Geometry: final body of the model. Coordinates: model frame, mm. Face numbers are marked on the shaded views. Give positions to 0.01 mm unless a question says otherwise; leave off trailing zeros. One line per question, with ' | ' between items. Start each with the question number.
Item 1: Pin query (flat end, axial travel): P1, Ø12, axis at x = 53.5, z = -242, coming from the +Y side; P2, Ø1.5, axis at x = 238.5, z = -43.5, coming from the -Y side. Return the tip coordinate at first contact, or that it passes through.
Item 2: Section A-A on y = 2.55. Give the number of separate pieces and of enclosed holes in the cut face, then the cut area to 3 significant figures.
Item 3: Material intervals for line 1 along X through (y, z) = (1.85, -227); line 2 along Z through (x, y) = (32.5, 1.3); line 3 along X through (y, z) = (1.8, -112), sorted ascending. Write a range as [from, to].
Item 4: Mould query, pull axis X, two halves, no side actions, for the marked faces 1 and 2. Classes: released by +X, released by -X, zero draft, split by the parting line, or undercut.
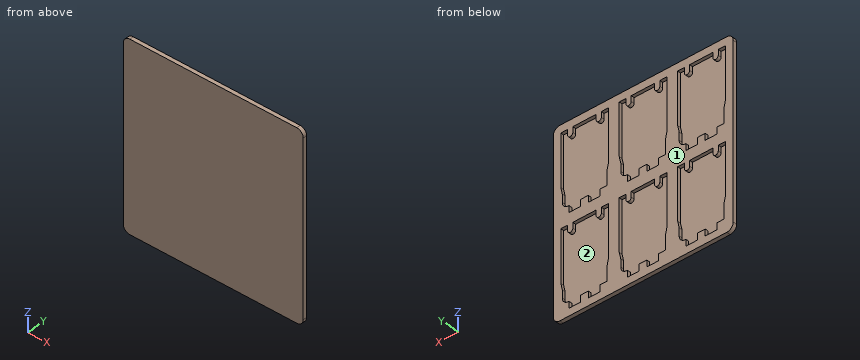
from build123d import *

# Parameters (mm, degrees)
BOSS_EXTRUDE1_DEPTH = 6
CUT_EXTRUDE1_DEPTH  = 5


with BuildPart() as part:
    # Sketch1 → Boss-Extrude1 (new body)
    with BuildSketch(Plane(origin=(0, 0, 0), x_dir=(1, 0, 0), z_dir=(0, 1, 0))):
        with BuildLine():
            Line((10, 0), (267, 0))
            ThreePointArc((267, 0), (274.071067812, 2.928932188), (277, 10))
            Line((277, 10), (277, 276))
            ThreePointArc((277, 276), (274.071067812, 283.071067812), (267, 286))
            Line((267, 286), (10, 286))
            ThreePointArc((10, 286), (2.928932188, 283.071067812), (0, 276))
            Line((0, 276), (0, 10))
            ThreePointArc((0, 10), (2.928932188, 2.928932188), (10, 0))
        make_face()
    extrude(amount=BOSS_EXTRUDE1_DEPTH)

    # Sketch2 → Cut-Extrude1 (cut)
    with BuildSketch(Plane(origin=(0, 6, 0), x_dir=(1, 0, 0), z_dir=(0, 1, 0))):
        with BuildLine():
            Line((12.062245302, 92), (14.402743297, 102.5))
            Line((14.402743297, 102.5), (14.402743297, 124.5))
            Line((14.402743297, 124.5), (25.102743297, 124.5))
            Line((25.102743297, 124.5), (25.102743297, 134.7))
            Line((25.102743297, 134.7), (43.102743297, 134.7))
            Line((43.102743297, 134.7), (43.102743297, 124.5))
            Line((43.102743297, 124.5), (54.902731898, 124.5))
            Line((54.902731898, 124.5), (54.902731898, 134.663480988))
            Line((54.902731898, 134.663480988), (72.902731898, 134.663480988))
            Line((72.902731898, 134.663480988), (72.902731898, 124.463480988))
            ThreePointArc((72.902731898, 124.463480988), (80.333662874, 121.834216678), (83.221747307, 114.5))
            Line((83.221747307, 114.5), (83.221747307, 102.5))
            Line((83.221747307, 102.5), (85.562245302, 91.74))
            Line((85.562245302, 91.74), (85.562245302, 12))
            Line((85.562245302, 12), (75.062245302, 12))
            Line((75.062245302, 12), (75.062245302, 20.5))
            ThreePointArc((75.062245302, 20.5), (71.062245302, 24.5), (67.062245302, 20.5))
            Line((67.062245302, 20.5), (67.062245302, 12))
            Line((67.062245302, 12), (31.062245302, 12))
            Line((31.062245302, 12), (31.062245302, 20.5))
            ThreePointArc((31.062245302, 20.5), (27.062245302, 24.5), (23.062245302, 20.5))
            Line((23.062245302, 20.5), (23.062245302, 12))
            Line((23.062245302, 12), (12.062245302, 12))
            Line((12.062245302, 12), (12.062245302, 92))
        make_face()
        with BuildLine():
            Line((102.062245302, 92), (104.402743297, 102.5))
            Line((104.402743297, 102.5), (104.402743297, 124.5))
            Line((104.402743297, 124.5), (115.102743297, 124.5))
            Line((115.102743297, 124.5), (115.102743297, 134.7))
            Line((115.102743297, 134.7), (133.102743297, 134.7))
            Line((133.102743297, 134.7), (133.102743297, 124.5))
            Line((133.102743297, 124.5), (144.902731898, 124.5))
            Line((144.902731898, 124.5), (144.902731898, 134.663480988))
            Line((144.902731898, 134.663480988), (162.902731898, 134.663480988))
            Line((162.902731898, 134.663480988), (162.902731898, 124.463480988))
            ThreePointArc((162.902731898, 124.463480988), (170.333662874, 121.834216678), (173.221747307, 114.5))
            Line((173.221747307, 114.5), (173.221747307, 102.5))
            Line((173.221747307, 102.5), (175.562245302, 91.74))
            Line((175.562245302, 91.74), (175.562245302, 12))
            Line((175.562245302, 12), (165.062245302, 12))
            Line((165.062245302, 12), (165.062245302, 20.5))
            ThreePointArc((165.062245302, 20.5), (161.062245302, 24.5), (157.062245302, 20.5))
            Line((157.062245302, 20.5), (157.062245302, 12))
            Line((157.062245302, 12), (121.062245302, 12))
            Line((121.062245302, 12), (121.062245302, 20.5))
            ThreePointArc((121.062245302, 20.5), (117.062245302, 24.5), (113.062245302, 20.5))
            Line((113.062245302, 20.5), (113.062245302, 12))
            Line((113.062245302, 12), (102.062245302, 12))
            Line((102.062245302, 12), (102.062245302, 92))
        make_face()
        with BuildLine():
            Line((192.062245302, 92), (194.402743297, 102.5))
            Line((194.402743297, 102.5), (194.402743297, 124.5))
            Line((194.402743297, 124.5), (205.102743297, 124.5))
            Line((205.102743297, 124.5), (205.102743297, 134.7))
            Line((205.102743297, 134.7), (223.102743297, 134.7))
            Line((223.102743297, 134.7), (223.102743297, 124.5))
            Line((223.102743297, 124.5), (234.902731898, 124.5))
            Line((234.902731898, 124.5), (234.902731898, 134.663480988))
            Line((234.902731898, 134.663480988), (252.902731898, 134.663480988))
            Line((252.902731898, 134.663480988), (252.902731898, 124.463480988))
            ThreePointArc((252.902731898, 124.463480988), (260.333662874, 121.834216678), (263.221747307, 114.5))
            Line((263.221747307, 114.5), (263.221747307, 102.5))
            Line((263.221747307, 102.5), (265.562245302, 91.74))
            Line((265.562245302, 91.74), (265.562245302, 12))
            Line((265.562245302, 12), (255.062245302, 12))
            Line((255.062245302, 12), (255.062245302, 20.5))
            ThreePointArc((255.062245302, 20.5), (251.062245302, 24.5), (247.062245302, 20.5))
            Line((247.062245302, 20.5), (247.062245302, 12))
            Line((247.062245302, 12), (211.062245302, 12))
            Line((211.062245302, 12), (211.062245302, 20.5))
            ThreePointArc((211.062245302, 20.5), (207.062245302, 24.5), (203.062245302, 20.5))
            Line((203.062245302, 20.5), (203.062245302, 12))
            Line((203.062245302, 12), (192.062245302, 12))
            Line((192.062245302, 12), (192.062245302, 92))
        make_face()
        with BuildLine():
            Line((102.062245302, 232), (104.402743297, 242.5))
            Line((104.402743297, 242.5), (104.402743297, 264.5))
            Line((104.402743297, 264.5), (115.102743297, 264.5))
            Line((115.102743297, 264.5), (115.102743297, 274.7))
            Line((115.102743297, 274.7), (133.102743297, 274.7))
            Line((133.102743297, 274.7), (133.102743297, 264.5))
            Line((133.102743297, 264.5), (144.902731898, 264.5))
            Line((144.902731898, 264.5), (144.902731898, 274.663480988))
            Line((144.902731898, 274.663480988), (162.902731898, 274.663480988))
            Line((162.902731898, 274.663480988), (162.902731898, 264.463480988))
            ThreePointArc((162.902731898, 264.463480988), (170.333662874, 261.834216678), (173.221747307, 254.5))
            Line((173.221747307, 254.5), (173.221747307, 242.5))
            Line((173.221747307, 242.5), (175.562245302, 231.74))
            Line((175.562245302, 231.74), (175.562245302, 152))
            Line((175.562245302, 152), (165.062245302, 152))
            Line((165.062245302, 152), (165.062245302, 160.5))
            ThreePointArc((165.062245302, 160.5), (161.062245302, 164.5), (157.062245302, 160.5))
            Line((157.062245302, 160.5), (157.062245302, 152))
            Line((157.062245302, 152), (121.062245302, 152))
            Line((121.062245302, 152), (121.062245302, 160.5))
            ThreePointArc((121.062245302, 160.5), (117.062245302, 164.5), (113.062245302, 160.5))
            Line((113.062245302, 160.5), (113.062245302, 152))
            Line((113.062245302, 152), (102.062245302, 152))
            Line((102.062245302, 152), (102.062245302, 232))
        make_face()
        with BuildLine():
            Line((192.062245302, 232), (194.402743297, 242.5))
            Line((194.402743297, 242.5), (194.402743297, 264.5))
            Line((194.402743297, 264.5), (205.102743297, 264.5))
            Line((205.102743297, 264.5), (205.102743297, 274.7))
            Line((205.102743297, 274.7), (223.102743297, 274.7))
            Line((223.102743297, 274.7), (223.102743297, 264.5))
            Line((223.102743297, 264.5), (234.902731898, 264.5))
            Line((234.902731898, 264.5), (234.902731898, 274.663480988))
            Line((234.902731898, 274.663480988), (252.902731898, 274.663480988))
            Line((252.902731898, 274.663480988), (252.902731898, 264.463480988))
            ThreePointArc((252.902731898, 264.463480988), (260.333662874, 261.834216678), (263.221747307, 254.5))
            Line((263.221747307, 254.5), (263.221747307, 242.5))
            Line((263.221747307, 242.5), (265.562245302, 231.74))
            Line((265.562245302, 231.74), (265.562245302, 152))
            Line((265.562245302, 152), (255.062245302, 152))
            Line((255.062245302, 152), (255.062245302, 160.5))
            ThreePointArc((255.062245302, 160.5), (251.062245302, 164.5), (247.062245302, 160.5))
            Line((247.062245302, 160.5), (247.062245302, 152))
            Line((247.062245302, 152), (211.062245302, 152))
            Line((211.062245302, 152), (211.062245302, 160.5))
            ThreePointArc((211.062245302, 160.5), (207.062245302, 164.5), (203.062245302, 160.5))
            Line((203.062245302, 160.5), (203.062245302, 152))
            Line((203.062245302, 152), (192.062245302, 152))
            Line((192.062245302, 152), (192.062245302, 232))
        make_face()
        with BuildLine():
            Line((12.062245302, 232), (14.402743297, 242.5))
            Line((14.402743297, 242.5), (14.402743297, 264.5))
            Line((14.402743297, 264.5), (25.102743297, 264.5))
            Line((25.102743297, 264.5), (25.102743297, 274.7))
            Line((25.102743297, 274.7), (43.102743297, 274.7))
            Line((43.102743297, 274.7), (43.102743297, 264.5))
            Line((43.102743297, 264.5), (54.902731898, 264.5))
            Line((54.902731898, 264.5), (54.902731898, 274.663480988))
            Line((54.902731898, 274.663480988), (72.902731898, 274.663480988))
            Line((72.902731898, 274.663480988), (72.902731898, 264.463480988))
            ThreePointArc((72.902731898, 264.463480988), (80.333662874, 261.834216678), (83.221747307, 254.5))
            Line((83.221747307, 254.5), (83.221747307, 242.5))
            Line((83.221747307, 242.5), (85.562245302, 231.74))
            Line((85.562245302, 231.74), (85.562245302, 152))
            Line((85.562245302, 152), (75.062245302, 152))
            Line((75.062245302, 152), (75.062245302, 160.5))
            ThreePointArc((75.062245302, 160.5), (71.062245302, 164.5), (67.062245302, 160.5))
            Line((67.062245302, 160.5), (67.062245302, 152))
            Line((67.062245302, 152), (31.062245302, 152))
            Line((31.062245302, 152), (31.062245302, 160.5))
            ThreePointArc((31.062245302, 160.5), (27.062245302, 164.5), (23.062245302, 160.5))
            Line((23.062245302, 160.5), (23.062245302, 152))
            Line((23.062245302, 152), (12.062245302, 152))
            Line((12.062245302, 152), (12.062245302, 232))
        make_face()
    extrude(amount=-CUT_EXTRUDE1_DEPTH, mode=Mode.SUBTRACT)


solid = part.part
Result sheet:
1) P1: stops at y = 1 | P2: stops at y = 0
2) separate pieces: 1 | enclosed holes: 6 | area: 29,300 mm²
3) line 1: x = [0, 12.06], [85.56, 102.06], [175.56, 192.06], [265.56, 277] | line 2: z = [-286, -274.7], [-152, -134.7], [-12, 0] | line 3: x = [0, 14.4], [83.22, 104.4], [173.22, 194.4], [263.22, 277]
4) face 1: zero draft | face 2: undercut
